CAD build for the part. Positions are in the model's coordinates, mm. Round coordinates to 2 decimals unless told otherwise and drop trailing zeros. Loops run counter-clockwise (first coordinate to the right, second up) from the corner with the lowest first, then second, coordinate; pieces in that order, holes last.
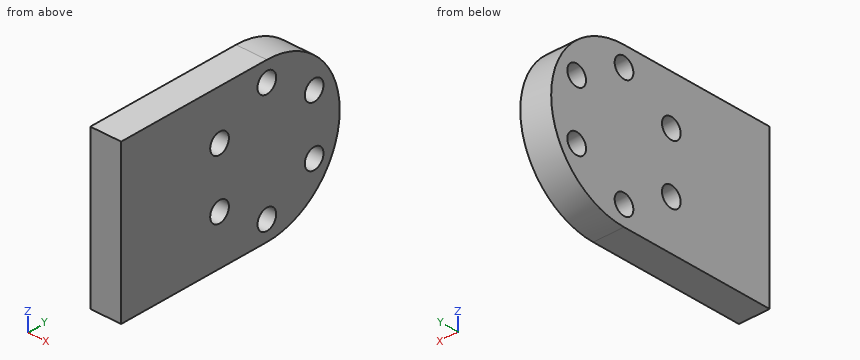
Autodesk Inventor part; units mm, degrees
ref_plane "Work Plane1" through (2.5019, 0, 0) normal (-1, 0, 0) x (0, 0, 1)
ref_plane "Work Plane2" through (0, -25.4, 0) normal (0, 0, -1) x (-1, 0, 0)
ref_plane "YZ Plane" through (0, 0, 0) normal (1, 0, 0) x (0, 1, 0)
sketch "Sketch1" plane through (0, 0, 0) normal (1, 0, 0) x (0, 1, 0)
  circle A0 centre (0, 0) radius 12.7
  circle A1 centre (0, 0) radius 6
  circle A2 centre (0, 9.525) radius 1.63
  circle A3 centre (8.2489, 4.7625) radius 1.63
  circle A4 centre (8.2489, -4.7625) radius 1.63
  circle A5 centre (0, -9.525) radius 1.63
  circle A6 centre (-8.2489, -4.7625) radius 1.63
  circle A7 centre (-8.2489, 4.7625) radius 1.63
  circle A8 centre (0, 0) radius 6
  circle A9 centre (0, 0) radius 3.2
  point P0 (0, 0.0001)
extrude "Extrusion1" add sketch "Sketch1" along normal blind 5.0038 contours A0 | A1 | A9
sketch "Sketch2" plane through (0, 0, 0) normal (-1, 0, 0) x (0, 0, 1)
  circle A0 centre (0, 0) radius 12.7
  line L0 (12.7, 0) -> (12.7, -25.4)
  line L1 (0, 0) -> (0, -12.7) construction
  line L2 (-12.7, 0) -> (-12.7, -25.4)
  line L3 (12.7, -25.4) -> (-12.7, -25.4)
  circle A1 centre (-9.525, 0) radius 1.63
  circle A2 centre (-4.7625, 8.2489) radius 1.63
  circle A3 centre (4.7625, 8.2489) radius 1.63
  circle A4 centre (4.7625, -8.2489) radius 1.63
  circle A5 centre (-4.7625, -8.2489) radius 1.63
  circle A6 centre (9.525, 0) radius 1.63
  circle A7 centre (0, 0) radius 12.7
  arc A8 (-12.7, 0) -> (12.7, 0) centre (0, 0) ccw
  dimension "d2" = 25.4
extrude "Extrusion2" add sketch "Sketch2" against normal blind 5.0038 contours L0 L3 L2 A0
ref_plane "Work Plane1" through (2.5019, 0, 0) normal (-1, 0, 0) x (0, 0, 1)
ref_plane "Work Plane2" through (0, -25.4, 0) normal (0, 0, -1) x (-1, 0, 0)
properties part number "thumb mount"
Item 1: Cut at B-B, the plane x = 3.3. Give the cut face in (y, z) (1 decimal).
Answers follow:
outline: (-25.4, -12.7) - (0, -12.7) arc R12.7 ccw to (0, 12.7) - (-25.4, 12.7) - close; hole circle Ø3.3 at (-8.2, -4.8); hole circle Ø3.3 at (-8.2, 4.8); hole circle Ø3.3 at (0, -9.5); hole circle Ø3.3 at (0, 9.5); hole circle Ø3.3 at (8.2, -4.8); hole circle Ø3.3 at (8.2, 4.8)
Item 2: Flat gauge pin, fed straight in: P1, Ø3, axis at y = 0, z = 9.525, coming from the -X side. Where does the tip first touch, or does it go through?
Answers follow:
P1: passes through
Item 3: Probe line 1 (Z direction, x = 3.5, y = 0) (3 decimals); line 2 (Y direction, x = 1.8, z = 6); line 3 (Y direction, x = 2.45, z = 6.25). List the from-to ranges inside material, lowest first.
Answers follow:
line 1: z = -12.7 to -11.155, -7.895 to 7.895, 11.155 to 12.7
line 2: y = -25.4 to -9.31, -7.19 to 7.19, 9.31 to 11.19
line 3: y = -25.4 to -8.92, -7.58 to 7.58, 8.92 to 11.06
Item 4: Cut at A-A, the plane y = -8.5. Give the cut face in (x, z).
Answers follow:
outline: (0, -12.7) - (5, -12.7) - (5, -6.37) - (0, -6.37) - close; (0, -3.15) - (5, -3.15) - (5, 3.15) - (0, 3.15) - close; (0, 6.37) - (5, 6.37) - (5, 12.7) - (0, 12.7) - close
